Geometry check sheet. Reference: the model listing, model coordinates, mm. Round coordinates to 2 decimals unless told otherwise and drop trailing zeros. Order: outer loops, then holes, each group sorted by start corner. A loop starts at its lowest first (then second) coordinate and runs counter-clockwise, first axis right, second up. Notation, with made-up numbers: (-14.75, 33.25) - (-9.75, 33.25) arc R32 ccw to (-9.75, 65.25) - close; hole circle Ø1 at (-36, -40). An arc over 180 degrees is marked (long way). Use a Markdown table: item, result. Add a question column.
(1) Thickness scan on line 1 along Y through (x, z) = (13.5, -13); line 2 along X through (y, z) = (142, 36.5); line 3 along Y through (x, z) = (19, 5). Record the ranges inside material, lowest first. Write a range as [from, to].
(2) Section check A-A on z = -26. Record the boundary of the cut face in (x, y), then the cut area to 3 significant figures.
(3) Section check B-B on x = 9.5. Record the boundary of the cut face in (y, z).
(4) Section check C-C on y = 147. Record the boundary of the cut face in (x, z).
```python
from build123d import *

# Parameters (mm, degrees)
EXTRUDE_1_DEPTH = 40
CHAMFER_1_SIZE  = 5
FILLET_1_R      = 5


with BuildPart() as part:
    # 草图1 → 凸台-拉伸1 (new, symmetric)
    with BuildSketch(Plane.XY):
        Polygon((0, 0), (0, 125), (13, 180), (20, 180), (20, 0), align=None)
    extrude(amount=EXTRUDE_1_DEPTH, both=True)

    # 倒角1
    chamfer_1_edges = [part.edges().sort_by_distance(p)[0] for p in [
        (10, 0, 40),
        (10, 0, -40),
        (0, 0, 0),
        (20, 0, 0),
    ]]
    chamfer(chamfer_1_edges, length=CHAMFER_1_SIZE)

    # 圆角1
    fillet_1_edges = [part.edges().sort_by_distance(p)[0] for p in [
        (0, 125, 0),
        (13, 180, 0),
    ]]
    fillet(fillet_1_edges, radius=FILLET_1_R)


solid = part.part
```
Check sheet entries:
| question | item | result |
|---|---|---|
| 1 | line 1 | y = [0, 178.61] |
| 1 | line 2 | x = [4.02, 20] |
| 1 | line 3 | y = [4, 180] |
| 2 | outline | (0, 5) - (5, 0) - (15, 0) - (20, 5) - (20, 180) - (16.96, 180) arc R5 ccw to (12.09, 176.15) - (0.13, 125.57) arc R5 ccw to (0, 124.42) - close |
| 2 | area | 3,210 mm2 |
| 3 | outline | (0, -35) - (5, -40) - (165.19, -40) - (165.19, 40) - (5, 40) - (0, 35) - close |
| 4 | outline | (5.2, -40) - (20, -40) - (20, 40) - (5.2, 40) - close |
